Design review of the part built by this model. Coordinates are the model's own, in mm. A direction names the side the tool comes from. Coordinates: 2 decimals unless noted, no trailing zeros. Write each loop counter-clockwise with the first axis right and the second up, starting at its lowest first coordinate (ties: lowest second). Pieces come first, ordered by that corner, then holes. Notation, with made-up numbers: (16.5, -24.75) - (31.5, -24.75) arc R26 cw to (31.5, -5.75) - close; hole circle Ø9 at (85.5, -29.5). An arc over 180 degrees is marked (long way). One line per item, written item: value.
from build123d import *

# Parameters (mm, degrees)
F0_W      = 127
F0_H      = 50.8
F1_DEPTH  = 38.1
F2_W      = 25.4
F2_H      = 25.4
F3_DEPTH  = 38.101
F5_DEPTH  = 38.101
F8_R      = 6.35
F7_R      = 6.35
F9_DEPTH  = 25.401
F6_W      = 25.4
F6_H      = 38.1
F10_DEPTH = 25.4
F12_DEPTH = 25.4


with BuildPart() as f1:
    # F0 (on Front) → F1 (new body)
    with BuildSketch(Plane.XZ):
        with Locations((14.029513, -1.326698)):
            Rectangle(F0_W, F0_H)
    extrude(amount=F1_DEPTH)

    # F2 (on face) → F3 (cut, through all)
    with BuildSketch(Plane.XZ.offset(38.1)):
        with Locations((-36.770487, 11.373302)):
            Rectangle(F2_W, F2_H)
        with Locations((64.829513, 11.373302)):
            Rectangle(F2_W, F2_H)
    extrude(amount=-F3_DEPTH, mode=Mode.SUBTRACT)

    # F4 (on face) → F5 (cut, through all)
    with BuildSketch(Plane.XZ.offset(38.1)):
        Polygon((-24.070487, 24.073302), (-24.070487, -1.326698), (-11.370487, 24.073302), align=None)
        Polygon((52.129513, 24.073302), (39.429513, 24.073302), (52.129513, -1.326698), align=None)
    extrude(amount=-F5_DEPTH, mode=Mode.SUBTRACT)

    # F8 (on face) + F7 (on face) → F9 (cut, through all)
    with BuildSketch(Plane.XY.offset(-1.326698)):
        with Locations((64.829513, -19.05)):
            Circle(F8_R)
    with BuildSketch(Plane.XY.offset(-1.326698)):
        with Locations((-36.770487, -19.05)):
            Circle(F7_R)
    extrude(amount=-F9_DEPTH, mode=Mode.SUBTRACT)

    # F6 (on face) → F10 (cut)
    with BuildSketch(Plane.XZ.offset(38.1)):
        with Locations((14.029513, 5.023302)):
            Rectangle(F6_W, F6_H)
    extrude(amount=-F10_DEPTH, mode=Mode.SUBTRACT)

    # F11 (on face) → F12 (join)
    with BuildSketch(Plane.YZ.offset(1.329513)):
        Polygon((-12.7, 24.073302), (-38.1, -14.026698), (-12.7, -14.026698), align=None)
    extrude(amount=F12_DEPTH)


solid = f1.part
1. Consider section B-B, the plane z = -16. Write out the cut boundary in (x, y), then the cut area to 3 significant figures.
Answer block:
outline: (-49.47, -38.1) - (77.53, -38.1) - (77.53, 0) - (-49.47, 0) - close; hole circle Ø12.7 at (-36.77, -19.05); hole circle Ø12.7 at (64.83, -19.05)
area: 4,590 mm^2
2. Mouldability with a two-part tool opening along Y and no side actions: class faces 1 (the face through (58.486, -18.771, -13.849)), 2 (the face through (59, -24, -1.327)), 3 (the face through (13, 0, -7)) as released by +Y, released by -Y, zero draft, split by the parting line, or undercut.
Answer block:
face 1: undercut
face 2: zero draft
face 3: released by +Y
3. Wall thickness on line 1 along X through (y, z) = (-19, -18); line 2 along X through (y, z) = (-15, -13); line 3 along Y through (x, z) = (-42, -24): over which ranges is each line inside the solid? List them lowest first.
Answer block:
line 1: x = -49.47 to -43.12, -30.42 to 58.48, 71.18 to 77.53
line 2: x = -49.47 to -41.66, -31.88 to 59.94, 69.72 to 77.53
line 3: y = -38.1 to -22.65, -15.45 to 0
4. Consider section C-C, the plane y = -11. Write out the cut boundary in (x, z).
Answer block:
outline: (-49.47, -26.73) - (77.53, -26.73) - (77.53, -1.33) - (52.13, -1.33) - (39.43, 24.07) - (-11.37, 24.07) - (-24.07, -1.33) - (-49.47, -1.33) - close
5. Insertion check: pin 1 Ø7.5 at (y, z) = (-21, 12) entering from -X; pin 2 Ø5 at (x, y) = (64, -24.5) entering from +Z; pin 3 Ø10 at (x, z) = (8, 17.5) entering from -Y. Each pin has a flat end and moves straight along its axis. Give the tip position at first contact, or say it passes through.
Answer block:
pin 1: stops at x = -19.28
pin 2: stops at z = -1.33
pin 3: stops at y = -20.42
6. Consider section D-D, the plane z = 9. Write out the cut boundary in (x, y).
Answer block:
outline: (-18.91, -38.1) - (1.33, -38.1) - (1.33, -22.75) - (26.73, -22.75) - (26.73, -38.1) - (46.97, -38.1) - (46.97, 0) - (-18.91, 0) - close
7. Consider section A-A, the plane y = -19.05. Write out the cut boundary in (x, z).
Answer block:
outline: (-49.47, -26.73) - (-43.12, -26.73) - (-43.12, -1.33) - (-49.47, -1.33) - close; (-30.42, -26.73) - (58.48, -26.73) - (58.48, -1.33) - (52.13, -1.33) - (39.43, 24.07) - (26.73, 24.07) - (26.73, 14.55) - (1.33, 14.55) - (1.33, 24.07) - (-11.37, 24.07) - (-24.07, -1.33) - (-30.42, -1.33) - close; (71.18, -26.73) - (77.53, -26.73) - (77.53, -1.33) - (71.18, -1.33) - close
8. For faces 4 (the face through (13.85, -25.22, 5.29)), 5 (the face through (-31, -24, -1.327)), 6 (the face through (14, -10, 24.073)), list the 3-axis set-ups (+Z, -Z, +X, -X, +Y, -Y) from which the entire face can be reached by the end or side of a thin tool; tool diameter is ignored.
Answer block:
face 4: +Z, -Y
face 5: +Z, -X, +Y, -Y
face 6: +Z, +X, -X, +Y, -Y
